Could you check a few things on this drawing? It's one solid part, dimensions in mm from its lowest x, y, z. Coordinates: 2 decimals unless noted, no trailing zeros. Write each loop counter-clockwise with the first axis right and the second up, starting at its lowest first coordinate (ties: lowest second). Pieces come first, ordered by that corner, then holes. Notation, with made-up numbers: M -5,48 L 16,48 A21 ccw 16,76 Z; hole C 55.25,38.25 d2. An arc over 180 degrees is marked long. Use a Markdown table: item, result.
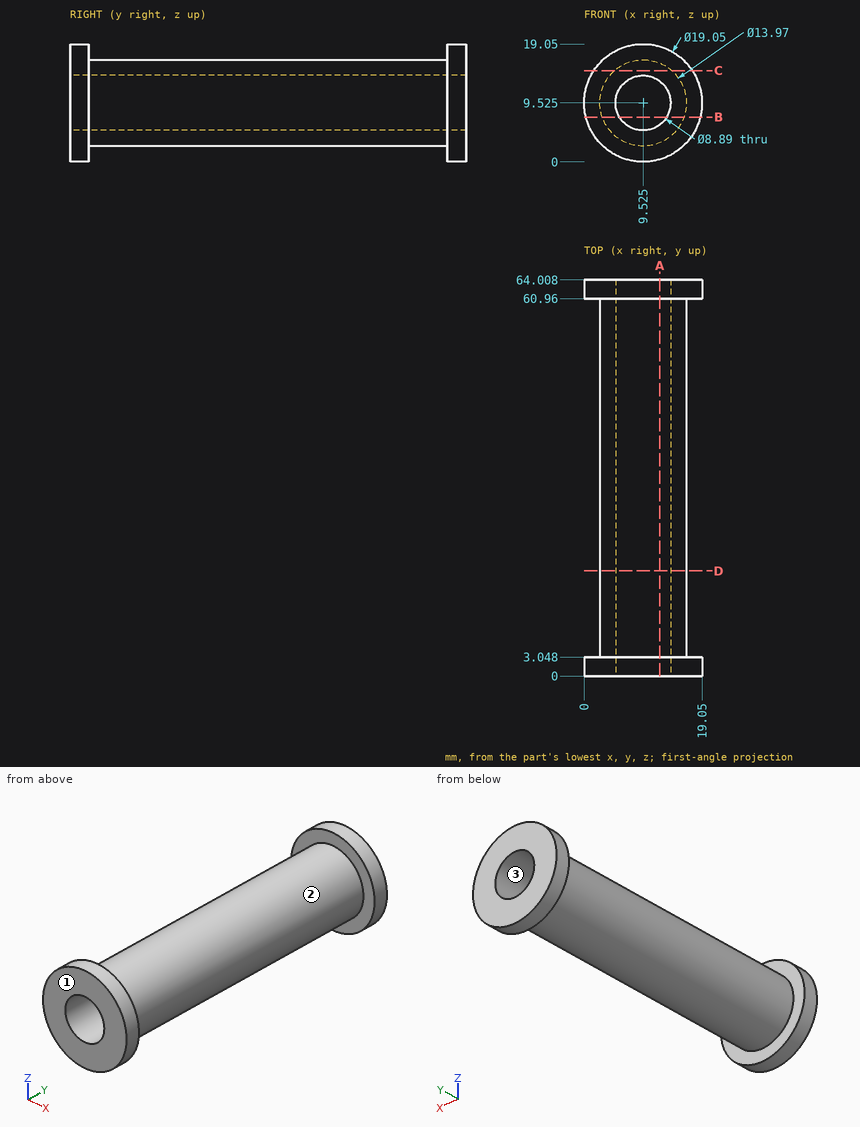
1. We'd pull the mould along Z, two halves only. Please class the marked faces 1, 2 and 3: +Z half, -Z half, draft (parallel to the pull), parting line (faces both ways), or undercut.
Answers follow:
| item | result |
|---|---|
| face 1 | draft |
| face 2 | parting line |
| face 3 | undercut |
2. Suppose I cut it at B-B on z = 7.25. Write out the boundary of the cut face in (x, y), and give its area (3 significant figures).
Answers follow:
| item | result |
|---|---|
| outline | M 0.28,0 L 5.71,0 L 5.71,64.01 L 0.28,64.01 L 0.28,60.96 L 2.92,60.96 L 2.92,3.05 L 0.28,3.05 Z; M 13.34,0 L 18.77,0 L 18.77,3.05 L 16.13,3.05 L 16.13,60.96 L 18.77,60.96 L 18.77,64.01 L 13.34,64.01 Z |
| area | 389 mm2 |
3. Suppose I cut it at A-A on x = 12.25. Write out the boundary of the cut face in (y, z).
Answers follow:
| item | result |
|---|---|
| outline | M 0,0.4 L 3.05,0.4 L 3.05,3.09 L 60.96,3.09 L 60.96,0.4 L 64.01,0.4 L 64.01,6.01 L 0,6.01 Z; M 0,13.04 L 64.01,13.04 L 64.01,18.65 L 60.96,18.65 L 60.96,15.96 L 3.05,15.96 L 3.05,18.65 L 0,18.65 Z |
4. Suppose I cut it at C-C on z = 14.75. Write out the boundary of the cut face in (x, y).
Answers follow:
| item | result |
|---|---|
| outline | M 1.56,0 L 17.49,0 L 17.49,3.05 L 14.16,3.05 L 14.16,60.96 L 17.49,60.96 L 17.49,64.01 L 1.56,64.01 L 1.56,60.96 L 4.89,60.96 L 4.89,3.05 L 1.56,3.05 Z |
5. I need wall thicknesses on probe 1 along Y at (x, z) = (7, 17); probe 2 along Z at (x, y) = (5.5, 48.5); probe 3 along Z at (x, y) = (11.75, 34). Which ranges of each line are inside material? Lowest first, please.
Answers follow:
| item | result |
|---|---|
| probe 1 | y = 0 to 3.05, 60.96 to 64.01 |
| probe 2 | z = 3.82 to 7.64, 11.41 to 15.23 |
| probe 3 | z = 2.9 to 5.68, 13.37 to 16.15 |
6. Suppose I cut it at D-D on y = 17. Write out the boundary of the cut face in (x, z) (3 decimals), and give its area (3 significant figures).
Answers follow:
| item | result |
|---|---|
| outline | C 9.525,9.525 d13.97; hole C 9.525,9.525 d8.89 |
| area | 91.2 mm2 |
7. Will these pins go through, and if not, where does the flat tip stop? pin 1 Ø1.5 at (y, z) = (56, 7) entering from +X; pin 2 Ø1 at (y, z) = (48.5, 12) entering from +X (3 decimals); pin 3 Ø3 at (x, y) = (4.5, 12.5) entering from -Z.
Answers follow:
| item | result |
|---|---|
| pin 1 | stops at x = 16.28 |
| pin 2 | stops at x = 16.225 |
| pin 3 | stops at z = 3.49 |
